Source: CAD feature listing. Evaluate the final solid. Frame: model axes, mm. Face numbers are marked on the shaded views. A direction names the side the tool comes from. Give positions to 0.01 mm unless a question says otherwise; leave off trailing zeros. Write each loop counter-clockwise with the first axis right and the second up, starting at its lowest first coordinate (ties: lowest second). Pieces come first, ordered by that corner, then holes.
```python
from build123d import *

# Parameters (mm, degrees)
F0_W     = 100
F0_H     = 45
F1_DEPTH = 10
F3_DEPTH = 45
F5_DEPTH = 122


with BuildPart() as f1:
    # F0 (on Top) → F1 (new body)
    with BuildSketch(Plane.XY):
        with Locations((-12.765671, -6.932852)):
            Rectangle(F0_W, F0_H)
    extrude(amount=F1_DEPTH)

    # F2 (on face) → F3 (join)
    with BuildSketch(Plane(origin=(0, 15.567148, 0), x_dir=(-1, 0, 0), z_dir=(0, 1, 0))):
        Polygon((12.765671, 39), (12.765671, 48), (-24.734329, 48), (-37.234329, 10), (12.765671, 10), (12.765671, 15), (0.765671, 15), (0.765671, 39), align=None)
        Polygon((50.265671, 48), (12.765671, 48), (12.765671, 39), (24.765671, 39), (24.765671, 15), (12.765671, 15), (12.765671, 10), (62.765671, 10), align=None)
    extrude(amount=-F3_DEPTH)

    # F4 (on face) → F5 (cut)
    with BuildSketch(Plane.YZ.offset(37.234329)):
        Polygon((-29.432852, 10), (-16.932852, 48), (-29.432852, 48), align=None)
        Polygon((15.567148, 48), (3.067148, 48), (15.567148, 10), align=None)
        Polygon((-0.932852, 27), (-6.932852, 27), (-12.932852, 27), (-12.932852, 15), (-0.932852, 15), align=None)
    extrude(amount=-F5_DEPTH, mode=Mode.SUBTRACT)


solid = f1.part
```
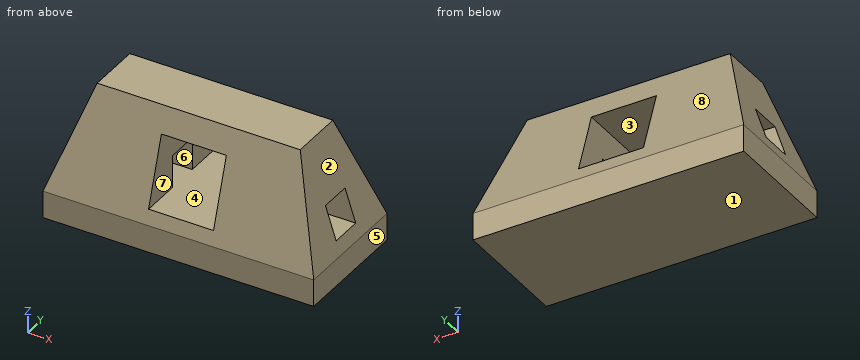
1. Cut plane C-C, the plane x = 7. Return the cut outline in (y, z), then the cut area to 3 significant figures.
2. Mould query, pull axis X, two halves, no side actions, for the marked faces 1, 2 and 3. Classes: +X half, -X half, draft (parallel to the pull), parting line (faces both ways), or undercut.
3. Cut plane D-D, the plane z = 29. Return the cut outline in (x, y), then the cut area to 3 significant figures.
4. Access query for the marked faces 4, 5, 6, 7 and 8. Directions: +Z, -Z, +X, -X, +Y, -Y. A direction counts if a zero-diameter tool reaches every point of the face in a straight line with its end or side. Return the directions, or none.
5. Cut plane B-B, the plane y = -2. Return the cut outline in (x, z).
6. Line query: L1, parallel to Z at x = -14, y = -10; L2, parallel to Z at x = 8, y = -7; L3, parallel to X at y = -9, z = 30. Output: solid intervals per line, ascending.
7. Contact query for flat-ended pins moving along their axis: P1, Ø19, axis at y = 0.5, z = 27.5, coming from the -X side; P2, Ø3.5, axis at x = 17, y = -5, coming from the -Z side; P3, Ø6, axis at x = -38.5, z = 23, coming from the -Y side; P4, Ø12, axis at y = 8.5, z = 17, coming from the -X side. Output: stop coordinate, or through.
8. Cut plane A-A, the plane x = -10.5. Return the cut outline in (y, z).
Response values:
1. outline: (-29.43, 0) - (15.57, 0) - (15.57, 10) - (3.07, 48) - (-16.93, 48) - (-29.43, 10) - close; hole (-12.93, 15) - (-0.93, 15) - (-0.93, 27) - (-12.93, 27) - close
1. area: 1,540 mm2
2. face 1: draft
2. face 2: +X half
2. face 3: undercut
3. outline: (-56.52, -23.18) - (-24.77, -23.18) - (-24.77, 9.32) - (-56.52, 9.32) - close; (-0.77, -23.18) - (30.98, -23.18) - (30.98, 9.32) - (-0.77, 9.32) - close
3. area: 2,060 mm2
4. face 4: none
4. face 5: +Z, -Z, +X, +Y, -Y
4. face 6: +X, -X
4. face 7: +Y, -Y
4. face 8: +Z, +X, -X, +Y
5. outline: (-62.77, 0) - (37.23, 0) - (37.23, 10) - (35.59, 15) - (-61.12, 15) - (-62.77, 10) - close; (-57.17, 27) - (-24.77, 27) - (-24.77, 39) - (-0.77, 39) - (-0.77, 27) - (31.64, 27) - (24.73, 48) - (-50.27, 48) - close
6. L1: z = 0 to 15, 39 to 48
6. L2: z = 0 to 15, 27 to 48
6. L3: x = -56.19 to -24.77, -0.77 to 30.66
7. P1: stops at x = -60.13
7. P2: stops at z = 0
7. P3: stops at y = -26.14
7. P4: stops at x = -62.44
8. outline: (-29.43, 0) - (15.57, 0) - (15.57, 10) - (13.92, 15) - (-27.79, 15) - (-29.43, 10) - close; (-19.89, 39) - (6.03, 39) - (3.07, 48) - (-16.93, 48) - close
